Design review of the part built by this model. Coordinates are the model's own, in mm. A direction names the side the tool comes from. Give positions to 0.01 mm unless a question says otherwise; leave off trailing zeros. Write each loop counter-clockwise with the first axis right and the second up, starting at its lowest first coordinate (ties: lowest second). Pieces come first, ordered by that corner, then holes. Notation, with made-up numbers: (-30, 17.5) -> (-19, 17.5) arc R19 ccw to (-19, 43.5) -> close; hole circle Ø1 at (75, 70.25). An arc over 180 degrees is marked (long way). Use CSV: the item, a comma, the result in double quotes.
```python
from build123d import *

# Parameters (mm, degrees)
ARROW_DEPTH = 1.27
SKETCH3_R   = 2.286
FLAG_DEPTH  = 6.35


with BuildPart() as part:
    # Sketch1 → dial base shape (revolve)
    with BuildSketch(Plane.XY, mode=Mode.PRIVATE) as dial_base_shape_sk:
        Polygon((0, -20.891058424), (0, -36.893058424), (12.7, -36.893058424), (12.7, -31.305058424), (3.175, -31.305058424), (3.175, -26.225058424), (12.7, -26.225058424), (12.7, -24.701058424), (15.24, -24.701058424), (15.24, -20.891058424), align=None)
    revolve(dial_base_shape_sk.sketch.rotate(Axis((0, -20.891058424, 0), (0, -1, 0)), 180), axis=Axis((0, -20.891058424, 0), (0, -1, 0)))

    # Sketch2 → arrow (add)
    with BuildSketch(Plane(origin=(0, -20.891058424, 0), x_dir=(1, 0, 0), z_dir=(0, 1, 0))):
        Polygon((0, 14.732), (-1.813922821, 8.382), (1.813922821, 8.382), align=None)
    extrude(amount=ARROW_DEPTH)

    # Sketch3 → flag (add)
    with BuildSketch(Plane.XZ.offset(36.893058424)):
        with Locations(Location((0, -9.854910999, 0), (0, 0, 180))):
            Circle(SKETCH3_R)
    extrude(amount=FLAG_DEPTH)


solid = part.part
```
(1) Take a section at B-B (x = 5.5). Write out the cut boundary in (y, z).
Established:
outline,"(-36.89, -11.45) -> (-31.31, -11.45) -> (-31.31, 11.45) -> (-36.89, 11.45) -> close; (-26.23, -11.45) -> (-24.7, -11.45) -> (-24.7, -14.21) -> (-20.89, -14.21) -> (-20.89, 14.21) -> (-24.7, 14.21) -> (-24.7, 11.45) -> (-26.23, 11.45) -> close"
(2) Take a section at D-D (z = 0). Write out the cut boundary in (x, y) (3 decimals).
Established:
outline,"(-15.24, -24.701) -> (-12.7, -24.701) -> (-12.7, -26.225) -> (-3.175, -26.225) -> (-3.175, -31.305) -> (-12.7, -31.305) -> (-12.7, -36.893) -> (12.7, -36.893) -> (12.7, -31.305) -> (3.175, -31.305) -> (3.175, -26.225) -> (12.7, -26.225) -> (12.7, -24.701) -> (15.24, -24.701) -> (15.24, -20.891) -> (-15.24, -20.891) -> close"
(3) Take a section at A-A (z = 6). Write out the cut boundary in (x, y), then the cut area to 3 significant figures.
Established:
outline,"(-14.01, -24.7) -> (-11.19, -24.7) -> (-11.19, -26.23) -> (11.19, -26.23) -> (11.19, -24.7) -> (14.01, -24.7) -> (14.01, -20.89) -> (-14.01, -20.89) -> close; (-11.19, -36.89) -> (11.19, -36.89) -> (11.19, -31.31) -> (-11.19, -31.31) -> close"
area,"266 mm2"
(4) For line 1 along Y through (x, z) = (9, 3.5); line 2 along Y through (x, z) = (1.5, -11.5); line 3 along Y through (x, z) = (-10.5, 10.5), list the stretches that pass through material, from the lowest coordinate up. Write a range as [from, to].
Established:
line 1,"y = [-36.89, -31.31], [-26.23, -20.89]"
line 2,"y = [-43.24, -31.31], [-26.23, -20.89]"
line 3,"y = [-24.7, -20.89]"
(5) Take a section at C-C (y = -27.25). Write out the cut boundary in (x, z) (3 decimals), then the cut area to 3 significant figures.
Established:
outline,"circle Ø6.35 at (0, 0)"
area,"31.7 mm2"
(6) Tool access review of faces 4 (the face through (-0.894, -20.265, -11.601)), 5 (the face through (-1.2, -40, -11.8)), 6 (the face through (0, -20, -8.382)): name each direction out of +Z, -Z, +X, -X, +Y, -Y from which nothing blocks a thin tool from reaching the whole face with its end or side.
Established:
face 4,"-Z, -X, +Y"
face 5,"-Y"
face 6,"+Z, +X, -X, +Y"
(7) Mouldability with a two-part tool opening along Y and no side actions: class faces 1 (the face through (0.92, -20.26, -11.51)), 2 (the face through (-3, -31.305, 3)), 3 (the face through (0, -36.893, 0)) as +Y half, -Y half, draft (parallel to the pull), parting line (faces both ways), or undercut.
Established:
face 1,"draft"
face 2,"undercut"
face 3,"-Y half"
(8) Clearance check with flat-ended pins moving along their axes: pin 1 (8 mm diameter, centred on y = -31.5, z = 7, fed in from -X); pin 2 (6 mm diameter, centred on y = -33, z = 5.5, fed in from -X); pin 3 (10 mm diameter, centred on x = -4, z = 3, fed in from -Y). State where each tip first meets the part, or that it passes through.
Established:
pin 1,"stops at x = -12.34"
pin 2,"stops at x = -12.45"
pin 3,"stops at y = -36.89"
